Can you work these out from the model? Positions are in its coordinate system, mm. Give positions to 0.01 mm unless a question says otherwise; leave off trailing zeros. Order: outer loops, then holes, each group sorted by start corner. A loop starts at its lowest first (then second) coordinate and runs counter-clockwise, first axis right, second up. Notation, with made-up numbers: (70.5, 37) - (92.5, 37) arc R16 ccw to (92.5, 56) - close; hole circle Ø3 at (15, 60). An arc over 180 degrees is marked (long way). Answer as a JSON object with one key per item and string values.
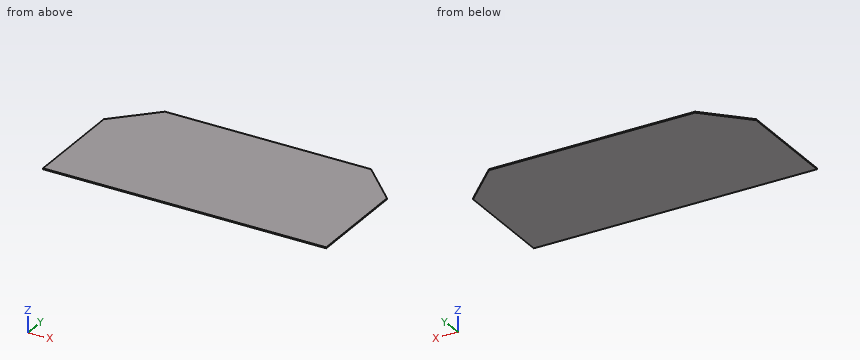
```python
from build123d import *

# Parameters (mm, degrees)
SKETCH1_W           = 80.15
SKETCH1_H           = 40.15
BOSS_EXTRUDE2_DEPTH = 0.28
CUT_EXTRUDE1_DEPTH  = 110.28
CUT_EXTRUDE2_DEPTH  = 10


with BuildPart() as part:
    # Sketch1 → Boss-Extrude2 (new body)
    with BuildSketch(Plane.XY):
        with Locations((13.610981812, 6.34266398)):
            Rectangle(SKETCH1_W, SKETCH1_H)
    extrude(amount=BOSS_EXTRUDE2_DEPTH)

    # Sketch3 → Cut-Extrude1 (cut)
    with BuildSketch(Plane.XY.offset(0.28)):
        Polygon((53.685981812, 26.41766398), (53.685981812, 15.51766398), (42.785981812, 26.41766398), align=None)
    extrude(amount=-CUT_EXTRUDE1_DEPTH, mode=Mode.SUBTRACT)

    # Sketch6 → Cut-Extrude2 (cut)
    with BuildSketch(Plane.XY.offset(0.28)):
        Polygon((-26.464018188, 26.41766398), (-26.464018188, 15.51766398), (-15.564018188, 26.41766398), align=None)
    extrude(amount=-CUT_EXTRUDE2_DEPTH, mode=Mode.SUBTRACT)


solid = part.part
```
Q1. I need wall thicknesses on L1, parallel to X at y = 19, z = 0.2; L2, parallel to X at y = 20.5, z = 0.1; L3, parallel to Y at x = 43.5, z = 0.15. Which ranges of each line are inside material? Lowest first, please.
Recorded:
{"L1": "x = -22.98 to 50.2", "L2": "x = -21.48 to 48.7", "L3": "y = -13.73 to 25.7"}
Q2. If we section it at A-A, the plane z = 0.2: Please give me the cut outline in (x, y), then the cut area to 3 significant figures.
Recorded:
{"outline": "(-26.46, -13.73) - (53.69, -13.73) - (53.69, 15.52) - (42.79, 26.42) - (-15.56, 26.42) - (-26.46, 15.52) - close", "area": "3,100 mm^2"}
Q3. If we section it at C-C, the plane x = 44.5: Please give me the cut outline in (y, z), then the cut area to 3 significant figures.
Recorded:
{"outline": "(-13.73, 0) - (24.7, 0) - (24.7, 0.28) - (-13.73, 0.28) - close", "area": "10.8 mm^2"}
Q4. If we section it at B-B, the plane y = 19: Please give me the cut outline in (x, z).
Recorded:
{"outline": "(-22.98, 0) - (50.2, 0) - (50.2, 0.28) - (-22.98, 0.28) - close"}
